Solid Edge part; units mm, degrees
sketch "Sketch1" plane through (0, 0, 0) normal (0, 0, 1) x (1, 0, 0)
  line L0 (-141.1152, 15.9486) -> (-41.1152, 15.9486)
  line L1 (-41.1152, 15.9486) -> (-41.1152, 115.9486)
  line L2 (-41.1152, 115.9486) -> (-141.1152, 115.9486)
  line L3 (-141.1152, 115.9486) -> (-141.1152, 15.9486)
extrude "Protrusion1" add sketch "Sketch1" along normal blind 5
sketch "Sketch2" plane through (-66.1152, 40.9486, 5) normal (0, 0, 1) x (1, 0, 0)
  circle A0 centre (-25, 25) radius 20
  dimension "D1" = 25
extrude "ExtrudedCutout_1" cut sketch "Sketch2" against normal blind 3
Design review of the part built by this model. Coordinates are the model's own, in mm. A direction names the side the tool comes from. Give positions to 0.01 mm unless a question says otherwise; leave off trailing zeros. Write each loop counter-clockwise with the first axis right and the second up, starting at its lowest first coordinate (ties: lowest second). Pieces come first, ordered by that corner, then holes. Notation, with made-up numbers: M 69,71 L 87,71 A18 cw 87,76 Z; hole C 79.5,6 d7. An arc over 180 degrees is marked long. Return JSON: item names as keys, results as strings. Group by question number.
Item 1: Take a section at A-A (y = 51.5). Give the boundary of the cut face in (x, z).
Item 2: The part is to be moulded in two halves that separate along Y. For faces 1 (the flat face through (-91, 66, 2)), 2 (the flat face through (-90, 115.949, 2)), 3 (the flat face through (-41.115, 65, 2)), say which applies: pulls with the +Y half, pulls with the -Y half, needs draft (parallel to the pull), parting line crosses it, or undercut.
Item 3: Tool access review of faces 4 (the cylindrical face through (-105.856, 79.466, 3.521)), 5 (the flat face through (-92, 15.949, 2)): name each direction out of +Z, -Z, +X, -X, +Y, -Y from which nothing blocks a thin tool from reaching the whole face with its end or side.
Item 4: Take a section at B-B (x = -100). Give the boundary of the cut face in (y, z).
Item 5: Clearance check with a flat-ended pin moving along its axis: pin 1 Ø12 at (x, y) = (-87, 66) entering from +Z. State where the tip first meets the part, or that it passes through.
Item 6: Wall thickness on line 1 along X through (y, z) = (65, 3.3); line 2 along Y through (x, z) = (-88, 4.2); line 3 along X through (y, z) = (81.5, 3.8): over which ranges is each line inside the solid? List them lowest first.
Item 7: Take a section at C-C (z = 2.85). Give the boundary of the cut face in (x, y).
Return value:
{
 "1": {"outline": "M -141.12,0 L -41.12,0 L -41.12,5 L -77.29,5 L -77.29,2 L -104.94,2 L -104.94,5 L -141.12,5 Z"},
 "2": {"face 1": "undercut", "face 2": "pulls with the +Y half", "face 3": "needs draft"},
 "3": {"face 4": "+Z", "face 5": "+Z, -Z, +X, -X, -Y"},
 "4": {"outline": "M 15.95,0 L 115.95,0 L 115.95,5 L 83.87,5 L 83.87,2 L 48.03,2 L 48.03,5 L 15.95,5 Z"},
 "5": {"pin 1": "stops at z = 2"},
 "6": {"line 1": "x = -141.12 to -111.09, -71.14 to -41.12", "line 2": "y = 15.95 to 46.19, 85.7 to 115.95", "line 3": "x = -141.12 to -103.69, -78.54 to -41.12"},
 "7": {"outline": "M -141.12,15.95 L -41.12,15.95 L -41.12,115.95 L -141.12,115.95 Z; hole C -91.12,65.95 d40"}
}
